Part print with two shaded views. Sizes in mm from the minimum x, y, z corner. Round coordinates to 2 decimals unless told otherwise and drop trailing zeros. Order: outer loops, then holes, each group sorted by start corner. A loop starts at its lowest first (then second) coordinate and runs counter-clockwise, first axis right, second up. Notation, with made-up numbers: (13.5, 78) -> (57.5, 78) arc R8 cw to (57.5, 93) -> close; hole circle Ø6 at (-40, 74). An arc over 180 degrees is marked (long way). Use a Markdown table: item, result. Add a question column.
Item 1: Slice it at C-C, the plane y = 16.5. Give the cut face in (x, z), plus the area to 3 significant figures.
Item 2: Pin check, flat tips, straight feed: pin 1 (1.6 mm diameter, centred on x = 16.5, z = 3, fed in from +Y); pin 2 (3 mm diameter, centred on y = 14.5, z = 11, fed in from +X); pin 3 (6.5 mm diameter, centred on y = 11, z = 13, fed in from -X). Stop position of each tip, or through.
Item 3: Slice it at A-A, the plane z = 14. Give the cut face in (x, y), plus the area to 3 significant figures.
Item 4: Two-plate mould, pull along Y, no slides. Class the marked faces 1 and 2: released by +Y, released by -Y, zero draft, split by the parting line, or undercut.
Item 5: Probe L1, parallel to X at y = 11, z = 3.5; L2, parallel to X at y = 13.75, z = 15.5; L3, parallel to Y at x = 13, z = 8.5. List the from-to ranges inside material, lowest first.
Item 6: Slice it at D-D, the plane x = 13.5. Give the cut face in (y, z).
Item 7: Slice it at B-B, the plane x = 5.5. Give the cut face in (y, z), plus the area to 3 significant figures.
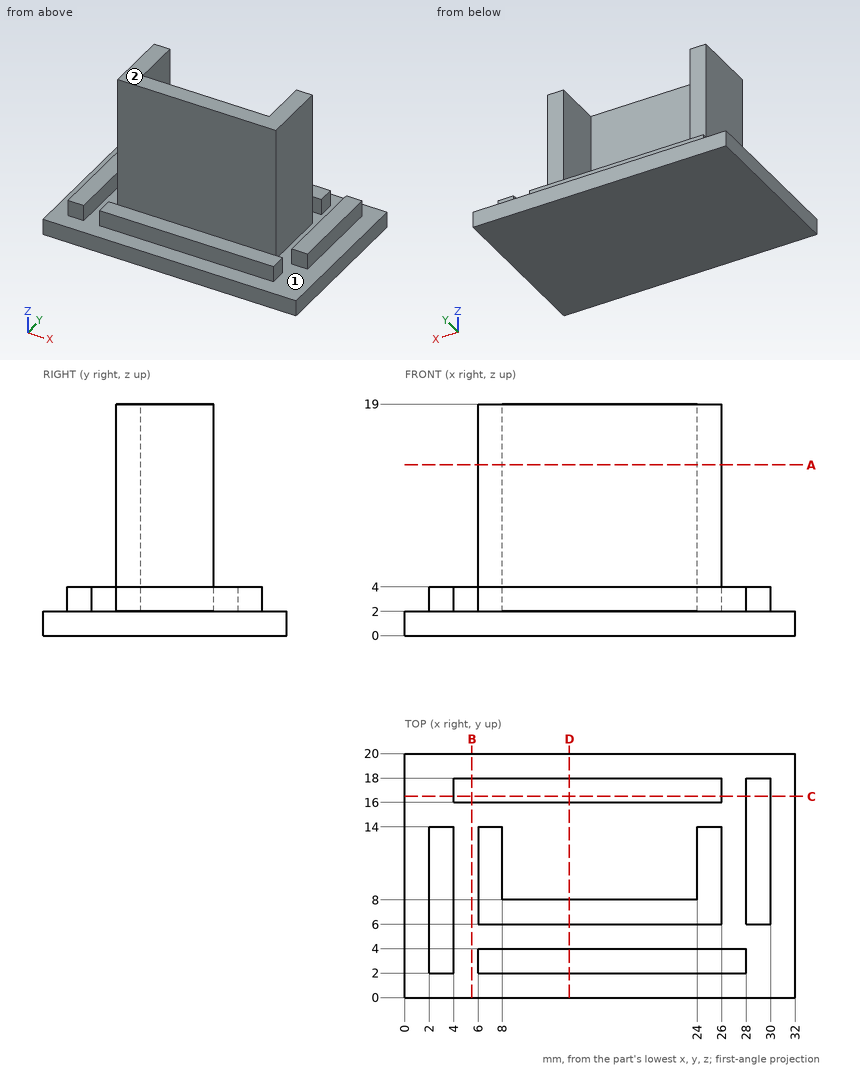
Check sheet entries:
| question | item | result |
|---|---|---|
| 1 | outline | (0, 0) -> (32, 0) -> (32, 2) -> (30, 2) -> (30, 4) -> (28, 4) -> (28, 2) -> (26, 2) -> (26, 4) -> (4, 4) -> (4, 2) -> (0, 2) -> close |
| 1 | area | 112 mm2 |
| 2 | pin 1 | y = 18 |
| 2 | pin 2 | x = 26 |
| 2 | pin 3 | x = 6 |
| 3 | outline | (6, 6) -> (26, 6) -> (26, 14) -> (24, 14) -> (24, 8) -> (8, 8) -> (8, 14) -> (6, 14) -> close |
| 3 | area | 64.0 mm2 |
| 4 | face 1 | undercut |
| 4 | face 2 | zero draft |
| 5 | L1 | 2 to 4, 6 to 8, 24 to 26, 28 to 30 |
| 5 | L2 | 6 to 8, 24 to 26 |
| 5 | L3 | 6 to 8 |
| 6 | outline | (0, 0) -> (20, 0) -> (20, 2) -> (18, 2) -> (18, 4) -> (16, 4) -> (16, 2) -> (8, 2) -> (8, 19) -> (6, 19) -> (6, 2) -> (4, 2) -> (4, 4) -> (2, 4) -> (2, 2) -> (0, 2) -> close |
| 7 | outline | (0, 0) -> (20, 0) -> (20, 2) -> (18, 2) -> (18, 4) -> (16, 4) -> (16, 2) -> (0, 2) -> close |
| 7 | area | 44.0 mm2 |
